The model under review builds one solid part; all positions refer to its coordinate system, in mm. Face numbers are marked on the shaded views. Round coordinates to 2 decimals unless told otherwise and drop trailing zeros. Order: outer loops, then holes, each group sorted by start corner. A loop starts at its lowest first (then second) coordinate and runs counter-clockwise, first axis right, second up.
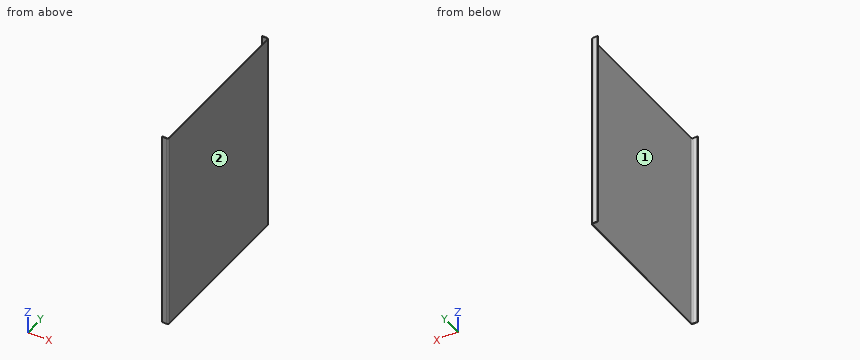
Autodesk Inventor part; units mm, degrees
ref_plane "YZ Plane" through (0, 0, 0) normal (1, 0, 0) x (0, 1, 0)
ref_plane "XZ Plane" through (0, 0, 0) normal (0, 1, 0) x (-1, 0, 0)
ref_plane "XY Plane" through (0, 0, 0) normal (0, 0, 1) x (1, 0, 0)
sketch "Náčrt2" plane through (0, 0, 0) normal (1, 0, 0) x (0, 1, 0)
  line L0 (800, 500) -> (0, 500)
  line L1 (0, 500) -> (0, -500)
  line L2 (0, -500) -> (800, -500)
  line L3 (800, -500) -> (800, 500)
  point P0 (0, 0)
  point P1 (0, 0)
  dimension "d0" = 1000
  dimension "d1" = 800
extrude "Vysunutí1" add sketch "Náčrt2" against normal blind 2.5
sketch "Náčrt3" plane through (0, 797.5, -500) normal (0, 1, 0) x (-1, 0, 0)
  line L0 (0, 1000) -> (0, 0)
  line L1 (0, 0) -> (31.5, 0)
  line L2 (31.5, 0) -> (31.5, 1000)
  line L3 (31.5, 1000) -> (0, 1000)
edge flange "Obruba1" height 31.5 angle 90 thickness 2.5 bend radius 6 thickness toward (0, 1, 0) relief tear relief width 2.5 relief depth 1.25 corner gap 2.5 corner form 0 edges at (-2.5, 800, 0) (-2.5, 0, 0) wall of the first edge with corners at (0, 797.5, 500) (0, 797.5, -500) (-31.5, 797.5, -500) (-31.5, 797.5, 500)
bend "Ohyb1"
corner "Roh1"
equation "\"d4\" = ŠířkaVýštipu"
equation "\"d5\" = HloubkaVýštipu"
equation "\"d6\" = MinimálníZbytek"
equation "\"d7\" = PoloměrOhybu"
equation "\"d11\" = VelikostRohovéhoVýštipu"
equation "\"d12\" = VelikostMezery"
equation "\"d13\" = VelikostJacobihoPoloměru"
equation "\"PoloměrOhybu\" = Tloušťka"
equation "\"ŠířkaVýštipu\" = Tloušťka"
equation "\"HloubkaVýštipu\" = 0.5 * Tloušťka"
equation "\"MinimálníZbytek\" = 2 * Tloušťka"
equation "\"PřechodovýPoloměr\" = PoloměrOhybu"
equation "\"VelikostJacobihoPoloměru\" = PoloměrOhybu"
equation "\"VelikostMezery\" = Tloušťka"
properties part number "DD_KVD_002_01" material "Nerezová ocel"
(1) Insertion check: pin 1 (8 mm diameter, centred on x = -7, y = 601.5, fed in from +Z); pin 2 (8 mm diameter, centred on y = 139, z = -317, fed in from -X). Each pin has a flat end and moves straight along its axis. Give the tip position at first contact, or say it passes through.
Data:
pin 1: passes through
pin 2: stops at x = -2.5
(2) To check wall thickness, follow probe 1 along Y at (x, z) = (-17, 82); probe 2 along Y at (x, z) = (-7.5, -404.5); probe 3 along X at (y, z) = (482, -181.5). State the ranges of each line that lie inside material, in increasing order.
Data:
probe 1: y = 0 to 2.5, 797.5 to 800
probe 2: y = 0.06 to 2.58, 797.42 to 799.94
probe 3: x = -2.5 to 0
(3) Consider section B-B (z = 379.5). Write out the cut boundary in (x, y), and give its area (3 significant figures).
Data:
outline: (-31.5, 0) - (-8.5, 0) arc R8.5 ccw to (0, 8.5) - (0, 791.5) arc R8.5 ccw to (-8.5, 800) - (-31.5, 800) - (-31.5, 797.5) - (-8.5, 797.5) arc R6 cw to (-2.5, 791.5) - (-2.5, 8.5) arc R6 cw to (-8.5, 2.5) - (-31.5, 2.5) - close
area: 2,130 mm2
(4) Consider section C-C (y = 681). Write out the cut boundary in (x, z).
Data:
outline: (-2.5, -500) - (0, -500) - (0, 500) - (-2.5, 500) - close
(5) Consider section A-A (x = -22.5). Write out the cut boundary in (y, z), and give its area (3 significant figures).
Data:
outline: (0, -500) - (2.5, -500) - (2.5, 500) - (0, 500) - close; (797.5, -500) - (800, -500) - (800, 500) - (797.5, 500) - close
area: 5,000 mm2
(6) Draft analysis for pull direction Y (two halves, no side actions). For the marked faces 1 and 2, state which applies: pulls with the +Y half, pulls with the -Y half, needs draft (parallel to the pull), parting line crosses it, or undercut.
Data:
face 1: undercut
face 2: needs draft
